from build123d import *

# Parameters (mm, degrees)
SKETCH_W        = 118.4
SKETCH_H        = 80
PAD_DEPTH       = 29
THICKNESS_T     = -1
SKETCH001_R     = 2
POCKET_DEPTH    = 29.001
SKETCH002_W     = 51
SKETCH002_H     = 40
POCKET001_DEPTH = 29.001
SKETCH003_R     = 2.05
SKETCH003_W     = 6.9
SKETCH003_H     = 2.95
POCKET002_DEPTH = 29.001
SKETCH004_R     = 4.05
SKETCH004_R_2   = 2.05
PAD001_DEPTH    = 12


with BuildPart() as part:
    # Sketch → Pad (new body)
    with BuildSketch(Plane.XY):
        Rectangle(SKETCH_W, SKETCH_H)
    extrude(amount=PAD_DEPTH)

    # Thickness
    thickness_openings = [part.faces().sort_by_distance(p)[0] for p in [
        (0, 0, 0),
    ]]
    offset(amount=THICKNESS_T, openings=thickness_openings)

    # Sketch001 → Pocket (cut, through all)
    with BuildSketch(Plane.XY):
        with Locations((53.5, 33)):
            Circle(SKETCH001_R)
        with Locations((53.5, -33)):
            Circle(SKETCH001_R)
        with Locations((-53.5, -33)):
            Circle(SKETCH001_R)
        with Locations((-53.5, 33)):
            Circle(SKETCH001_R)
    extrude(amount=POCKET_DEPTH, mode=Mode.SUBTRACT)

    # Sketch002 → Pocket001 (cut, through all)
    with BuildSketch(Plane.XY):
        with Locations((3.5, 1)):
            Rectangle(SKETCH002_W, SKETCH002_H)
    extrude(amount=POCKET001_DEPTH, mode=Mode.SUBTRACT)

    # Sketch003 → Pocket002 (cut, through all)
    with BuildSketch(Plane.XY):
        with Locations((49, 17.6)):
            Circle(SKETCH003_R)
        with Locations((49, 5)):
            Circle(SKETCH003_R)
        with Locations((49, -7.6)):
            Circle(SKETCH003_R)
        with Locations((49, -20.2)):
            Circle(SKETCH003_R)
        with Locations((38.2, -33)):
            Circle(SKETCH003_R)
        with Locations((-46.3, 16.14)):
            Rectangle(SKETCH003_W, SKETCH003_H)
        with Locations((-46.3, -1.76)):
            Rectangle(SKETCH003_W, SKETCH003_H)
        with Locations((-46.3, -19.66)):
            Rectangle(SKETCH003_W, SKETCH003_H)
    extrude(amount=POCKET002_DEPTH, mode=Mode.SUBTRACT)

    # Sketch004 (on DatumPlane) → Pad001 (join)
    with BuildSketch(Plane.XY.offset(28)):
        with Locations((49, 17.6)):
            Circle(SKETCH004_R)
        with Locations((49, 17.6)):
            Circle(SKETCH004_R_2, mode=Mode.SUBTRACT)
        with Locations((49, 5)):
            Circle(SKETCH004_R)
        with Locations((49, 5)):
            Circle(SKETCH004_R_2, mode=Mode.SUBTRACT)
        with Locations((49, -7.6)):
            Circle(SKETCH004_R)
        with Locations((49, -7.6)):
            Circle(SKETCH004_R_2, mode=Mode.SUBTRACT)
        with Locations((49, -20.2)):
            Circle(SKETCH004_R)
        with Locations((49, -20.2)):
            Circle(SKETCH004_R_2, mode=Mode.SUBTRACT)
        with Locations((38.2, -33)):
            Circle(SKETCH004_R)
        with Locations((38.2, -33)):
            Circle(SKETCH004_R_2, mode=Mode.SUBTRACT)
    extrude(amount=-PAD001_DEPTH)


solid = part.part
The listing builds one solid part. Answer for the finished solid, in the listing's coordinates (mm). A direction names the side the tool comes from. Coordinates: 2 decimals unless noted, no trailing zeros. Write each loop counter-clockwise with the first axis right and the second up, starting at its lowest first coordinate (ties: lowest second). Pieces come first, ordered by that corner, then holes. Notation, with made-up numbers: M 54,-1 L 63,-1 A16 cw 63,17 Z; hole C 87.25,47.5 d11. An arc over 180 degrees is marked long. Put each result on its own line as item: value. Start each with the question number.
1. Which of the six approach directions +Z, -Z, +X, -X, +Y, -Y give full straight-line access (tool end or side, diameter ignored) to faces 1 (the cylindrical face through (46.95, 5.09, 22.41)), 2 (the flat face through (51, -9, 16))?
2. A cutting plane is placed at D-D on x = 6. Write down the section's boundary in (y, z).
3. A cutting plane is placed at B-B on x = -53.5. Write down the section's boundary in (y, z).
4. Flat-ended cylindrical pins translate along their axes: P1, Ø3, axis at x = -35, y = 7.5, coming from the -Z side; P2, Ø2.5, axis at x = 51, y = 19, coming from the -Z side. Find the tip coordinate at first contact, or state that the pin passes through.
5. A cutting plane is placed at A-A on z = 18.5. Count the separate pieces of the cut face and the enclosed holes in it, then the cut area to 3 significant figures.
6. A cutting plane is placed at C-C on y = 33. Write down the section's boundary in (x, z).
7. For a pull along Y with two mould halves and no side action, classify faces 3 (the cylindrical face through (46.015, -4.863, 22.084)), 4 (the cylindrical face through (-53.934, 31.048, 28.493)), 5 (the flat face through (-59.2, -1, 14)) as pulls with the +Y half, pulls with the -Y half, needs draft (parallel to the pull), parting line crosses it, or undercut.
8. Consider line 1 (X direction, y = 33, z = 28.35); line 2 (Y direction, x = 38, z = 19); line 3 (Y direction, x = 53.5, z = 28.4). Determine where each line is inside the solid, lowest interval first. Write a range as from..to.
Resolved:
1. face 1: +Z, -Z
1. face 2: -Z
2. outline: M -40,0 L -39,0 L -39,28 L -19,28 L -19,29 L -40,29 Z; M 21,28 L 39,28 L 39,0 L 40,0 L 40,29 L 21,29 Z
3. outline: M -40,0 L -39,0 L -39,28 L -35,28 L -35,29 L -40,29 Z; M -31,28 L 31,28 L 31,29 L -31,29 Z; M 35,28 L 39,28 L 39,0 L 40,0 L 40,29 L 35,29 Z
4. P1: stops at z = 28
4. P2: stops at z = 16
5. separate pieces: 6
5. enclosed holes: 6
5. area: 584 mm2
6. outline: M -59.2,0 L -58.2,0 L -58.2,28 L -55.5,28 L -55.5,29 L -59.2,29 Z; M -51.5,28 L 51.5,28 L 51.5,29 L -51.5,29 Z; M 55.5,28 L 58.2,28 L 58.2,0 L 59.2,0 L 59.2,29 L 55.5,29 Z
7. face 3: undercut
7. face 4: undercut
7. face 5: needs draft
8. line 1: x = -59.2..-55.5, -51.5..51.5, 55.5..59.2
8. line 2: y = -40..-39, -37.05..-35.04, -30.96..-28.95, 39..40
8. line 3: y = -40..-35, -31..31, 35..40
